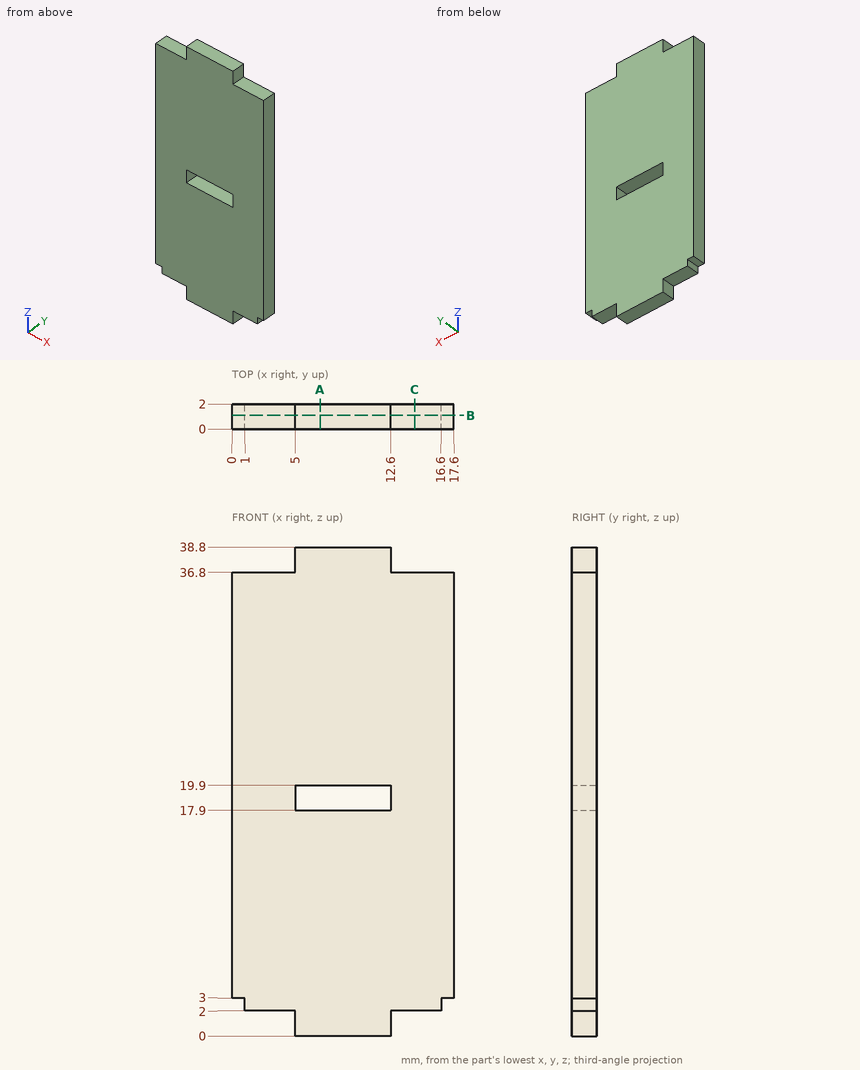
Geometry: see drawing. Coordinates: mm, zero at the bounding-box minimum. Give positions to 0.01 mm unless a question says otherwise; leave off trailing zeros. Order: outer loops, then holes, each group sorted by start corner. A loop starts at its lowest first (then second) coordinate and runs counter-clockwise, first axis right, second up. Notation, with made-up numbers: (-30.5, -10) - (16.5, -10) arc R20 ccw to (16.5, 0) - close; hole circle Ø10 at (64, 75.25). An arc over 180 degrees is marked (long way). One line per item, written item: value.
1. Line query: probe 1 along Z at (x, y) = (9, 1.55); probe 2 along Z at (x, y) = (16, 1.6). Output: solid intervals per line, ascending.
Determined:
probe 1: 0 to 17.9, 19.9 to 38.8
probe 2: 2 to 36.8
2. Cut plane C-C, the plane x = 14.5. Output: boundary loops of the cut face in (y, z).
Determined:
outline: (0, 2) - (2, 2) - (2, 36.8) - (0, 36.8) - close
3. Pin query (flat end, axial travel): pin 1 Ø1 at (y, z) = (1, 19) entering from -X; pin 2 Ø1 at (y, z) = (1.5, 37.5) entering from -X; pin 3 Ø1 at (x, y) = (4, 1.5) entering from -Z; pin 4 Ø0.6 at (y, z) = (0.5, 38) entering from +X. Return the tip coordinate at first contact, or that it passes through.
Determined:
pin 1: x = 0
pin 2: x = 5
pin 3: z = 2
pin 4: x = 12.6
4. Cut plane A-A, the plane x = 7. Output: boundary loops of the cut face in (y, z).
Determined:
outline: (0, 0) - (2, 0) - (2, 17.9) - (0, 17.9) - close; (0, 19.9) - (2, 19.9) - (2, 38.8) - (0, 38.8) - close
5. Cut plane B-B, the plane y = 1.1. Output: boundary loops of the cut face in (x, z), and give its area (3 significant figures).
Determined:
outline: (0, 3) - (1, 3) - (1, 2) - (5, 2) - (5, 0) - (12.6, 0) - (12.6, 2) - (16.6, 2) - (16.6, 3) - (17.6, 3) - (17.6, 36.8) - (12.6, 36.8) - (12.6, 38.8) - (5, 38.8) - (5, 36.8) - (0, 36.8) - close; hole (5, 17.9) - (12.6, 17.9) - (12.6, 19.9) - (5, 19.9) - close
area: 626 mm2
